Autodesk Inventor part; units mm, degrees
ref_plane "YZ Plane" through (0, 0, 0) normal (1, 0, 0) x (0, 1, 0)
ref_plane "XZ Plane" through (0, 0, 0) normal (0, 1, 0) x (-1, 0, 0)
ref_plane "XY Plane" through (0, 0, 0) normal (0, 0, 1) x (1, 0, 0)
sketch "Sketch1" plane through (0, 0, 0) normal (0, 1, 0) x (-1, 0, 0)
  circle A0 centre (0, 0) radius 2.5
  circle A1 centre (0, 0) radius 3.5
  dimension "PenetrationUpstreamInnerDiameter" = 5
  dimension "PenetrationUpstreamThickness" = 1
sketch "Sketch2" plane through (0, 0, 0) normal (0, 0, 1) x (1, 0, 0)
  line L0 (-7.62, 10.16) -> (-71.12, 10.16)
  line L1 (0, 0) -> (0, 2.54)
  arc A0 (0, 2.54) -> (-7.62, 10.16) centre (-7.62, 2.54) ccw
  dimension "PenetrationUpstreamLength" = 63.5
  dimension "d14" = 90
  dimension "PenetrationUpstreamDistanceFromWallToCentre" = 10.16
  dimension "StraightBit" = 2.54
sweep "Sweep2" add profiles "Sketch1" path "Sketch2"
equation "\"StraightBit\" = 0.25 * PenetrationUpstreamDistanceFromWallToCentre"
properties part number "PenetrationUpstream"
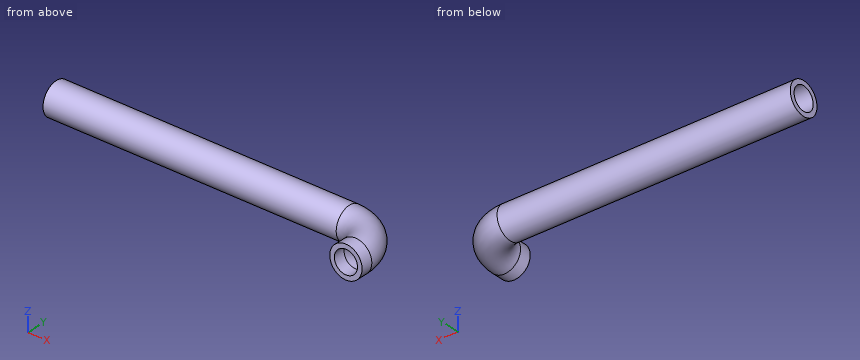
The listing builds one solid part. Answer for the finished solid, in the listing's coordinates (mm). Coordinates: 2 decimals unless noted, no trailing zeros. Write each loop counter-clockwise with the first axis right and the second up, starting at its lowest first coordinate (ties: lowest second). Pieces come first, ordered by that corner, then holes. Notation, with made-up numbers: (66, 55) - (116, 55) arc R15 cw to (116, 72) - close; hole circle Ø5 at (64.5, 18). An arc over 180 degrees is marked (long way). Return JSON: item names as keys, results as strings. Group by question number.
Q1. Find the intervals of material crossed by line 1 along Z through (x, y) = (0, 1.2); line 2 along Y through (x, z) = (-11, 1.5); line 3 along Y through (x, z) = (-29, 2), in increasing order. Write a range as [from, to].
Q2. The part is cut by section A-A on z = 1.5. Write down the section's boundary in (x, y), and give its area (3 significant figures).
Q3. Flat-ended cylindrical pins translate along their axes: pin 1 Ø1.5 at (y, z) = (2.5, 1) entering from -X; pin 2 Ø1 at (y, z) = (6, 2) entering from -X; pin 3 Ø5 at (x, y) = (-22, 4) entering from +Z; pin 4 Ø3 at (x, z) = (-34.5, 1.5) entering from -Y. Find the tip coordinate at first contact, or state that the pin passes through.
Q4. The part is cut by section B-B on x = -11.5. Write down the section's boundary in (y, z).
Evaluation:
{
 "1": {"line 1": "z = [-3.5, -2.5], [2.5, 3.5]", "line 2": "y = [7, 8.16], [12.16, 13.32]", "line 3": "y = [7.29, 8.66], [11.66, 13.03]"},
 "2": {"outline": "(-71.12, 7) - (-7.62, 7) arc R4.46 cw to (-3.16, 2.54) - (-3.16, 0) - (-2, 0) - (-2, 2.54) arc R5.62 ccw to (-7.62, 8.16) - (-71.12, 8.16) - close; (-71.12, 12.16) - (-7.62, 12.16) arc R9.62 cw to (2, 2.54) - (2, 0) - (3.16, 0) - (3.16, 2.54) arc R10.78 ccw to (-7.62, 13.32) - (-71.12, 13.32) - close", "area": "181 mm2"},
 "3": {"pin 1": "stops at x = -3.5", "pin 2": "stops at x = -5.19", "pin 3": "passes through", "pin 4": "stops at y = 6.66"},
 "4": {"outline": "circle Ø7 at (10.16, 0); hole circle Ø5 at (10.16, 0)"}
}
